Read the model definition and answer for the solid it produces. Units are mm, in the model's axes. Face numbers are marked on the shaded views. A direction names the side the tool comes from. Coordinates: 2 decimals unless noted, no trailing zeros. Loops run counter-clockwise (first coordinate to the right, second up) from the corner with the lowest first, then second, coordinate; pieces in that order, holes last.
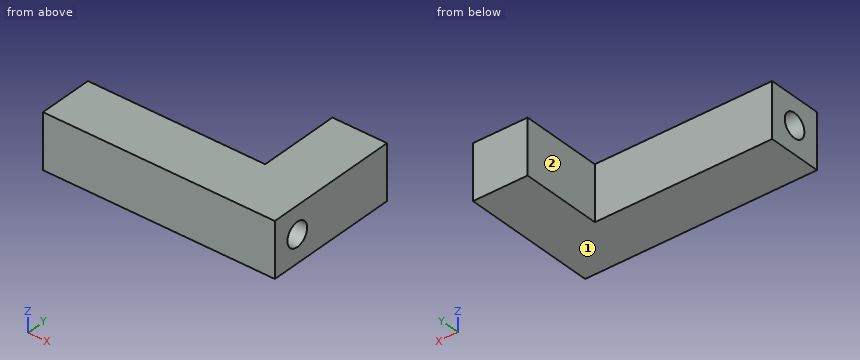
Solid Edge part; units mm, degrees
sketch "Sketch1" plane through (0, 0, 0) normal (0, 0, 1) x (1, 0, 0)
  line L0 (13, 4) -> (-13, 4)
  line L1 (-13, 4) -> (-13, -4)
  line L2 (-13, -4) -> (13, -4)
  line L3 (13, -4) -> (21, -4)
  line L4 (21, -4) -> (21, 16)
  line L5 (21, 16) -> (13, 16)
  line L6 (13, 16) -> (13, 4)
extrude "Protrusion1" add sketch "Sketch1" against normal blind 8
sketch "Sketch2" plane through (-13, 0, -4) normal (-1, 0, 0) x (0, 0, 1)
  circle A0 centre (0, 0) radius 1.75
extrude "Extrusionsausschnitt_1" cut sketch "Sketch2" against normal blind 38.1
Q1. Which of the six approach directions +Z, -Z, +X, -X, +Y, -Y give full straight-line access (tool end or side, diameter ignored) to the marked faces 1 and 2?
Findings below:
face 1: -Z, +X, -X, +Y, -Y
face 2: +Z, -Z, -X, +Y
Q2. A cutting plane is placed at C-C (x = 9). Give the vertices of the cut face in (y, z), then the cut area to 3 significant figures.
Findings below:
outline: (-4, -8) - (4, -8) - (4, 0) - (-4, 0) - close; hole circle Ø3.5 at (0, -4)
area: 54.4 mm2
Q3. Flat-ended cylindrical pins translate along their axes: pin 1 Ø4 at (y, z) = (11, -4) entering from -X; pin 2 Ø2 at (x, z) = (1, -6.5) entering from +Y. Find the tip coordinate at first contact, or state that the pin passes through.
Findings below:
pin 1: stops at x = 13
pin 2: stops at y = 4
Q4. A cutting plane is placed at B-B (y = 0). Give the vertices of the cut face in (x, z), then the cut area to 3 significant figures.
Findings below:
outline: (-13, -8) - (21, -8) - (21, -5.75) - (-13, -5.75) - close; (-13, -2.25) - (21, -2.25) - (21, 0) - (-13, 0) - close
area: 153 mm2
Q5. A cutting plane is placed at A-A (z = -4). Give the vertices of the cut face in (x, y).
Findings below:
outline: (-13, -4) - (21, -4) - (21, -1.75) - (-13, -1.75) - close; (-13, 1.75) - (21, 1.75) - (21, 16) - (13, 16) - (13, 4) - (-13, 4) - close
Q6. A cutting plane is placed at D-D (z = -6.75). Give the vertices of the cut face in (x, y), then the cut area to 3 significant figures.
Findings below:
outline: (-13, -4) - (21, -4) - (21, 16) - (13, 16) - (13, 4) - (-13, 4) - close
area: 368 mm2
Q7. Straight lines are drawn through the part: probe 1 along Y at (x, z) = (-3, -4); probe 2 along X at (y, z) = (12, -1); probe 3 along Y at (x, z) = (-2.5, -2.5). For each, find the intervals that lie inside material, in ascending order.
Findings below:
probe 1: y = -4 to -1.75, 1.75 to 4
probe 2: x = 13 to 21
probe 3: y = -4 to -0.9, 0.9 to 4
